from build123d import *

# Parameters (mm, degrees)
BOSS_EXTRUDE1_DEPTH                            = 5.5
DRAFT1_ANGLE                                   = -15
BOSS_EXTRUDE3_DEPTH                            = 5.5
SKETCH11_W                                     = 36
SKETCH11_H                                     = 45
BOSS_EXTRUDE4_DEPTH                            = 7
SKETCH12_R                                     = 1.65
CUT_EXTRUDE1_DEPTH                             = 10
CSK_FOR_M4_FLAT_HEAD_MACHINE_SCREW1_AT_2_COUNT = 2
CSK_FOR_M4_FLAT_HEAD_MACHINE_SCREW1_AT_2_PITCH = 26
CSK_FOR_M4_FLAT_HEAD_MACHINE_SCREW1_AT_3_COUNT = 2
CSK_FOR_M4_FLAT_HEAD_MACHINE_SCREW1_AT_3_PITCH = 35
CSK_FOR_M4_FLAT_HEAD_MACHINE_SCREW1_AT_4_COUNT = 2
CSK_FOR_M4_FLAT_HEAD_MACHINE_SCREW1_AT_4_PITCH = 43.600458713
FILLET1_R                                      = 5
CHAMFER1_SIZE                                  = 3
CUT_EXTRUDE2_DEPTH                             = 7


with BuildPart() as part:
    # Sketch1 → Boss-Extrude1 (new body)
    with BuildSketch(Plane(origin=(0, 0, 0), x_dir=(1, 0, 0), z_dir=(0, 1, 0))):
        Polygon((-5.798989873, -18.601010127), (-14, -10.4), (-14, 10.4), (-5.798989873, 18.601010127), (5.798989873, 18.601010127), (14, 10.4), (14, -10.4), (5.798989873, -18.601010127), align=None)
    extrude(amount=BOSS_EXTRUDE1_DEPTH)

    # Draft1
    draft1_faces = [part.faces().sort_by_distance(p)[0] for p in [
        (0, 2.75, 18.601010127),
        (-9.899494937, 2.75, 14.500505063),
        (-14, 2.75, 0),
        (9.899494937, 2.75, 14.500505063),
        (-9.899494937, 2.75, -14.500505063),
        (0, 2.75, -18.601010127),
        (9.899494937, 2.75, -14.500505063),
        (14, 2.75, 0),
    ]]
    draft(draft1_faces, Plane(origin=(0, 0, 0), x_dir=(0, 0, -1), z_dir=(0, -1, 0)), DRAFT1_ANGLE)

    # Sketch10 → Boss-Extrude3 (add)
    with BuildSketch(Plane.XZ):
        with BuildLine():
            Line((-14, -10.4), (14, -10.4))
            Line((14, -10.4), (5.798989873, -18.601010127))
            ThreePointArc((5.798989873, -18.601010127), (0, -21.00303038), (-5.798989873, -18.601010127))
            Line((-5.798989873, -18.601010127), (-14, -10.4))
        make_face()
        with BuildLine():
            Line((-14, 10.4), (14, 10.4))
            Line((14, 10.4), (5.798989873, 18.601010127))
            ThreePointArc((5.798989873, 18.601010127), (0, 21.00303038), (-5.798989873, 18.601010127))
            Line((-5.798989873, 18.601010127), (-14, 10.4))
        make_face()
    extrude(amount=-BOSS_EXTRUDE3_DEPTH)

    # Cut-Sweep1: sweep along a path in Sketch9
    with BuildLine(Plane.XZ) as cut_sweep1_path:
        Line((-20.807897552, -3.592102448), (-14, -10.4))
        Line((-14, -10.4), (-5.798989873, -18.601010127))
        ThreePointArc((-5.798989873, -18.601010127), (0, -21.00303038), (5.798989873, -18.601010127))
        Line((5.798989873, -18.601010127), (14, -10.4))
        Line((14, -10.4), (20.807897552, -3.592102448))
    # Sketch7 → Cut-Sweep1 (sweep, cut)
    with BuildSketch(Plane(origin=(14, 0, -10.4), x_dir=(-0.7071067811865477, 0, 0.7071067811865474), z_dir=(-0.7071067811865474, 0, -0.7071067811865477))):
        with BuildLine():
            Line((-3.263557389, 5.754), (1.376270031, 5.754))
            ThreePointArc((1.376270031, 5.754), (1.477025905, 5.704312701), (1.498942611, 5.594129981))
            Line((1.498942611, 5.594129981), (-0.159697719, -0.596))
            Line((-0.159697719, -0.596), (-3.263557389, -0.596))
            Line((-3.263557389, -0.596), (-3.263557389, 5.754))
        make_face()
    cut_sweep1 = sweep(path=cut_sweep1_path.line, mode=Mode.SUBTRACT)

    # Mirror1: Cut-Sweep1 across plane
    add(cut_sweep1.mirror(Plane.XY), mode=Mode.SUBTRACT)

    # Sketch11 → Boss-Extrude4 (add)
    with BuildSketch(Plane(origin=(0, 5.5, 0), x_dir=(1, 0, 0), z_dir=(0, 1, 0))):
        Rectangle(SKETCH11_W, SKETCH11_H)
    extrude(amount=BOSS_EXTRUDE4_DEPTH)

    # Sketch12 → Cut-Extrude1 (cut)
    with BuildSketch(Plane.XZ.offset(-5.5)):
        with Locations(Location((-13, 17.5, 0), (0, 0, 270))):
            Circle(SKETCH12_R)
        with Locations(Location((13, 17.5, 0), (0, 0, 90))):
            Circle(SKETCH12_R)
        with Locations(Location((13, -17.5, 0), (0, 0, 270))):
            Circle(SKETCH12_R)
        with Locations(Location((-13, -17.5, 0), (0, 0, 90))):
            Circle(SKETCH12_R)
    extrude(amount=-CUT_EXTRUDE1_DEPTH, mode=Mode.SUBTRACT)

    # Sketch3 → CSK for M4 Flat Head Machine Screw1 (revolve, cut)
    with BuildSketch(Plane(origin=(13, 5.5, -17.5), x_dir=(0, 0, -1), z_dir=(1, 0, 0))):
        Polygon((0, 0), (0, 4.351936393), (2.25, 3), (2.25, 2.45), (4.7, 0), align=None)
    csk_for_m4_flat_head_machine_screw1 = revolve(axis=Axis((13, -0.85, -17.5), (0, 1, 0)), mode=Mode.SUBTRACT)

    # CSK for M4 Flat Head Machine Screw1 at 2: CSK for M4 Flat Head Machine Screw1 ×2
    with Locations(*[(-i * CSK_FOR_M4_FLAT_HEAD_MACHINE_SCREW1_AT_2_PITCH, 0, 0) for i in range(1, CSK_FOR_M4_FLAT_HEAD_MACHINE_SCREW1_AT_2_COUNT)]):
        add(csk_for_m4_flat_head_machine_screw1, mode=Mode.SUBTRACT)

    # CSK for M4 Flat Head Machine Screw1 at 3: CSK for M4 Flat Head Machine Screw1 ×2
    with Locations(*[(0, 0, i * CSK_FOR_M4_FLAT_HEAD_MACHINE_SCREW1_AT_3_PITCH) for i in range(1, CSK_FOR_M4_FLAT_HEAD_MACHINE_SCREW1_AT_3_COUNT)]):
        add(csk_for_m4_flat_head_machine_screw1, mode=Mode.SUBTRACT)

    # CSK for M4 Flat Head Machine Screw1 at 4: CSK for M4 Flat Head Machine Screw1 ×2
    with Locations(*[Vector(-0.5963240013375937, 0, 0.8027438479544529) * (i * CSK_FOR_M4_FLAT_HEAD_MACHINE_SCREW1_AT_4_PITCH) for i in range(1, CSK_FOR_M4_FLAT_HEAD_MACHINE_SCREW1_AT_4_COUNT)]):
        add(csk_for_m4_flat_head_machine_screw1, mode=Mode.SUBTRACT)

    # Fillet1
    fillet1_edges = [part.edges().sort_by_distance(p)[0] for p in [
        (18, 9, 22.5),
        (18, 9, -22.5),
        (-18, 9, -22.5),
        (-18, 9, 22.5),
    ]]
    fillet(fillet1_edges, radius=FILLET1_R)

    # Sketch13 → Cut-Revolve1 (revolve, cut)
    with BuildSketch(Plane(origin=(0, 0, 0), x_dir=(0, 0, -1), z_dir=(1, 0, 0)), mode=Mode.PRIVATE) as cut_revolve1_sk:
        Polygon((0, 14.8), (0, -4.2), (7, -4.2), (7, 2.8), (7, 21.459689624), (0, 21.459689624), align=None)
    revolve(cut_revolve1_sk.sketch.rotate(Axis((0, -5.116386004, 0), (0, 1, 0)), 180), axis=Axis((0, -5.116386004, 0), (0, 1, 0)), mode=Mode.SUBTRACT)

    # Chamfer1
    chamfer1_edges = [part.edges().sort_by_distance(p)[0] for p in [
        (0, 0, -7),
    ]]
    chamfer(chamfer1_edges, length=CHAMFER1_SIZE)

    # Sketch14 → Cut-Extrude2 (cut)
    with BuildSketch(Plane(origin=(0, 12.5, 0), x_dir=(1, 0, 0), z_dir=(0, 1, 0))):
        with BuildLine():
            Line((18, -17.5), (18, 17.5))
            ThreePointArc((18, 17.5), (16.535533906, 21.035533906), (13, 22.5))
            Line((13, 22.5), (-13, 22.5))
            ThreePointArc((-13, 22.5), (-16.535533906, 21.035533906), (-18, 17.5))
            Line((-18, 17.5), (-18, -17.5))
            ThreePointArc((-18, -17.5), (-16.535533906, -21.035533906), (-13, -22.5))
            Line((-13, -22.5), (13, -22.5))
            ThreePointArc((13, -22.5), (16.535533906, -21.035533906), (18, -17.5))
        make_face()
    extrude(amount=-CUT_EXTRUDE2_DEPTH, mode=Mode.SUBTRACT)


solid = part.part
Geometry check sheet. Reference: the model listing, model coordinates, mm. Give positions to 0.01 mm unless a question says otherwise; leave off trailing zeros. Loops run counter-clockwise (first coordinate to the right, second up) from the corner with the lowest first, then second, coordinate; pieces in that order, holes last. Notation, with made-up numbers: M 19,38.5 L 45,38.5 A16 ccw 45,50.5 Z; hole C 44.25,12.5 d5. An arc over 180 degrees is marked long. Write each question's results on one line, items separated by ' | '.
1) Section check C-C, the plane y = 2.25. Record the boundary of the cut face in (x, z), plus the area to 3 significant figures.
Answers follow:
outline: M -13.4,-10.15 L -5.37,-18.17 A7.6 ccw 5.37,-18.17 L 13.4,-10.15 L 13.4,10.15 L 5.37,18.17 A7.6 ccw -5.37,18.17 L -13.4,10.15 Z; hole C 0,0 d15.5 | area: 689 mm2
2) Section check B-B, the plane x = 0. Record the boundary of the cut face in (y, z), plus the area to 3 significant figures.
Answers follow:
outline: M 0,-21 L 5.5,-19.53 L 5.5,-7 L 3,-7 L 0,-10 Z; M 0,10 L 3,7 L 5.5,7 L 5.5,19.53 L 0,21 Z | area: 137 mm2
3) Release check for a two-part mould opening along X. For faces 1 (the face through (-2.681, 4.267, 6.466)), 2 (the face through (-6, 5.5, -5)), 3 (the face through (-13.273, 2.711, 0.146)) record: +X half, -X half, draft (parallel to the pull), parting line (faces both ways), or undercut.
Answers follow:
face 1: undercut | face 2: draft | face 3: -X half
4) Gauge pin test, flat ends, axial feed: pin 1 (3 mm diameter, centred on x = 6, y = 1, fed in from -Z); pin 2 (11 mm diameter, centred on x = 0, z = 0, fed in from +Y); pin 3 (1.5 mm diameter, centred on x = 4, z = -6.5, fed in from -Y). Record the tip position at first contact, or that the pin passes through.
Answers follow:
pin 1: z = -19.44 | pin 2: through | pin 3: y = 1.62
5) Section check A-A, the plane z = 0. Record the boundary of the cut face in (x, y), plus the area to 3 significant figures.
Answers follow:
outline: M -14,0 L -10,0 L -7,3 L -7,5.5 L -12.53,5.5 Z; M 7,3 L 10,0 L 14,0 L 12.53,5.5 L 7,5.5 Z | area: 59.9 mm2
6) Section check D-D, the plane z = -11. Record the boundary of the cut face in (x, y).
Answers follow:
outline: M -13.4,0 L 13.4,0 L 11.32,5.5 L -11.32,5.5 Z
7) Thickness scan on line 1 (X direction, y = 4.5, z = 0); line 2 (X direction, y = 3.65, z = 0); line 3 (Z direction, x = -5.75, y = 2.1). Record the ranges inside material, lowest first.
Answers follow:
line 1: -12.79 to -7, 7 to 12.79 | line 2: -13.02 to -7, 7 to 13.02 | line 3: -17.85 to -5.42, 5.42 to 17.85
